Part model, mm, in its own coordinate system. Coordinates: 2 decimals unless noted, no trailing zeros. Write each loop counter-clockwise with the first axis right and the second up, starting at its lowest first coordinate (ties: lowest second). Pieces come first, ordered by that corner, then holes. Notation, with made-up numbers: (42, -39) - (53, -39) arc R32 ccw to (53, -10) - close; hole circle Ø1 at (-12, 89.25). An arc over 180 degrees is marked (long way). Use a Markdown table: item, result.
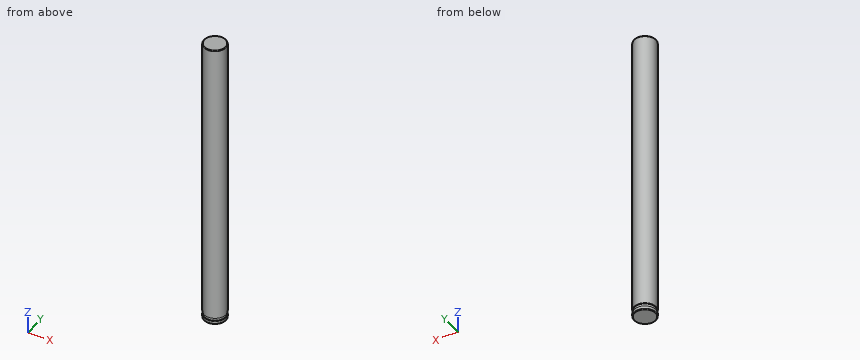
```python
from build123d import *

# Parameters (mm, degrees)
SKETCH1_R           = 1.5
BOSS_EXTRUDE1_DEPTH = 40
FILLET1_R           = 0.1
FILLET2_R           = 0.1
SKETCH2_W           = 0.148162506
SKETCH2_H           = 0.4


with BuildPart() as part:
    # Sketch1 → Boss-Extrude1 (new body)
    with BuildSketch(Plane.XY):
        Circle(SKETCH1_R)
    extrude(amount=BOSS_EXTRUDE1_DEPTH)

    # Fillet1
    fillet1_edges = [part.edges().sort_by_distance(p)[0] for p in [
        (-1.5, 0, 40),
    ]]
    fillet(fillet1_edges, radius=FILLET1_R)

    # Fillet2
    fillet2_edges = [part.edges().sort_by_distance(p)[0] for p in [
        (-1.5, 0, 0),
    ]]
    fillet(fillet2_edges, radius=FILLET2_R)

    # Sketch2 → Cut-Revolve1 (revolve, cut)
    with BuildSketch(Plane(origin=(0, 0, 0), x_dir=(1, 0, 0), z_dir=(0, 1, 0))):
        with Locations((-1.508482483, -0.675553033)):
            Rectangle(SKETCH2_W, SKETCH2_H)
    revolve(axis=Axis((0, 0, 0), (0, 0, 1)), mode=Mode.SUBTRACT)


solid = part.part
```
Item 1: Drill centre lines: probe 1 along Y at (x, z) = (0.1, 8); probe 2 along Y at (x, z) = (-0.55, 5); probe 3 along X at (y, z) = (-1.2, 37.5). Where is each one in solid material? Low to high.
From the geometry:
| item | result |
|---|---|
| probe 1 | -1.5 to 1.5 |
| probe 2 | -1.4 to 1.4 |
| probe 3 | -0.9 to 0.9 |
Item 2: Band-saw the part on A-A, the plane z = 11. Give the cut face in (x, y).
From the geometry:
| item | result |
|---|---|
| outline | circle Ø3 at (0, 0) |
Item 3: Drop a flat-ended pin along its axis: P1, Ø1.5, axis at x = -0.5, z = 11.5, coming from the +Y side. Give the stop position or say it passes through.
From the geometry:
| item | result |
|---|---|
| P1 | y = 1.5 |
